Source: CAD feature listing. Evaluate the final solid. Frame: model axes, mm. A direction names the side the tool comes from. Give positions to 0.01 mm unless a question says otherwise; leave off trailing zeros. Order: outer loops, then holes, each group sorted by start corner. A loop starts at its lowest first (then second) coordinate and runs counter-clockwise, first axis right, second up. Notation, with made-up numbers: M -39,64.25 L -4,64.25 A25 ccw -4,88.25 Z; hole C -1.75,-25 d7. An arc over 180 degrees is marked long. Answer in a Markdown table with one row per item. Add a question column.
(1) Section query A-A, the plane z = 3. Return loops of the section in (x, y) (3 decimals), plus the area to 3 significant figures.
(2) Section query C-C, the plane z = 20.5. Return loops of the section in (x, y) (3 decimals), plus the area to 3 significant figures.
(3) Mould query, pull axis X, two halves, no side actions, for faces 5 (the face through (-63.5, 0, 13)), 6 (the face through (-26.261, 19.547, 22.471)), 7 (the face through (0, 17, -25.4)), 8 (the face through (76.2, 0, 25)). Classes: pulls with the +X half, pulls with the -X half, needs draft (parallel to the pull), parting line crosses it, or undercut.
(4) Section query D-D, the plane x = 36. Return loops of the section in (y, z).
(5) Section query B-B, the plane z = 30. Count the separate pieces of the cut face and the enclosed holes in it, plus the area to 3 significant figures.
(6) Set-up query: faces 1 (the face through (-60.324, 0.332, 12.878)), 2 (the face through (-21.368, 21.274, 30.185)), 3 (the face through (35.67, -12.6, 28.53)), 4 (the face through (-35.67, 12.6, 28.53)). Return all of +Z, -Z, +X, -X, +Y, -Y with unobstructed straight access to the full face (end or side cutting, diameter ignored); none if empty.
(7) Material intervals for line 1 along Z through (x, y) = (-64.5, 15) (3 decimals); line 2 along X through (y, z) = (-20, 29); line 3 along X through (y, z) = (19, 10.5), sorted ascending.
(8) Pin query (flat end, axial travel): P1, Ø2.5, axis at x = 24.4, y = 20.32, coming from the +Z side; P2, Ø6.5, axis at x = 24.4, y = -20.32, coming from the -Z side; P3, Ø5, axis at x = -8.5, z = -5.5, coming from the -Y side. Return the tip coordinate at first contact, or that it passes through.
from build123d import *

# Parameters (mm, degrees)
SKETCH1_W                        = 152.4
SKETCH1_H                        = 63.5
BOSS_EXTRUDE1_DEPTH              = 25.4
BOSS_EXTRUDE2_DEPTH              = 9.525
BOSS_EXTRUDE3_DEPTH              = 6.35
CUT_EXTRUDE1_DEPTH               = 87.36933773
SKETCH5_R                        = 25.4
BOSS_EXTRUDE4_DEPTH              = 25.4
CUT_EXTRUDE2_DEPTH               = 103.242887894
F_7_16_20_TAPPED_HOLE2_OUTLINE_W = 4.96062
F_7_16_20_TAPPED_HOLE2_OUTLINE_H = 9.52526547
SKETCH13_R                       = 3.175
CUT_EXTRUDE3_DEPTH               = 3.175
F_10_32_TAPPED_HOLE1_D           = 4.0386
F_10_32_TAPPED_HOLE1_DEPTH       = 12.0396
F_10_32_TAPPED_HOLE1_TIP         = 1.213317848
FILLET1_R                        = 3.175
SKETCH16_W                       = 12.7
SKETCH16_H                       = 6.35
CUT_EXTRUDE4_DEPTH               = 106.159144277
CHAMFER1_SIZE                    = 9.525
CHAMFER2_SIZE                    = 9.525


# Read off the part's stored shape, not the designer's step: 7/16-20 Tapped Hole2
with BuildPart() as part:
    # Sketch1 → Boss-Extrude1 (new body)
    with BuildSketch(Plane.XY):
        Rectangle(SKETCH1_W, SKETCH1_H)
    extrude(amount=BOSS_EXTRUDE1_DEPTH)

    # Sketch2 → Boss-Extrude2 (add)
    with BuildSketch(Plane.XY.offset(25.4)):
        with BuildLine():
            Line((-57.15, 31.75), (-76.2, 31.75))
            Line((-76.2, 31.75), (-76.2, -31.75))
            Line((-76.2, -31.75), (-57.15, -31.75))
            ThreePointArc((-57.15, -31.75), (-65.65738686, 0), (-57.15, 31.75))
        make_face()
        with BuildLine():
            Line((57.15, 31.75), (76.2, 31.75))
            Line((76.2, 31.75), (76.2, -31.75))
            Line((76.2, -31.75), (57.15, -31.75))
            ThreePointArc((57.15, -31.75), (65.65738686, 0), (57.15, 31.75))
        make_face()
    extrude(amount=BOSS_EXTRUDE2_DEPTH)

    # Sketch3 → Boss-Extrude3 (add)
    with BuildSketch(Plane.XY.offset(25.4)):
        with BuildLine():
            ThreePointArc((0, 31.75), (-6.499067792, 31.272316494), (-12.858450657, 29.849532861))
            ThreePointArc((-12.858450657, 29.849532861), (-20.139715933, 27.86213325), (-27.51768912, 26.270878114))
            ThreePointArc((-27.51768912, 26.270878114), (-29.380205079, 25.48503317), (-30.748971212, 23.997418552))
            ThreePointArc((-30.748971212, 23.997418552), (-35.717260564, 12.431977761), (-37.689378393, 0))
            ThreePointArc((-37.689378393, 0), (-35.717260564, -12.431977761), (-30.748971212, -23.997418552))
            ThreePointArc((-30.748971212, -23.997418552), (-29.380205079, -25.48503317), (-27.51768912, -26.270878114))
            ThreePointArc((-27.51768912, -26.270878114), (-20.139715933, -27.86213325), (-12.858450657, -29.849532861))
            ThreePointArc((-12.858450657, -29.849532861), (-6.499067792, -31.272316494), (0, -31.75))
            ThreePointArc((0, -31.75), (6.499067792, -31.272316494), (12.858450657, -29.849532861))
            ThreePointArc((12.858450657, -29.849532861), (20.139715933, -27.86213325), (27.51768912, -26.270878114))
            ThreePointArc((27.51768912, -26.270878114), (29.380205079, -25.48503317), (30.748971212, -23.997418552))
            ThreePointArc((30.748971212, -23.997418552), (35.717260564, -12.431977761), (37.689378393, 0))
            ThreePointArc((37.689378393, 0), (35.717260564, 12.431977761), (30.748971212, 23.997418552))
            ThreePointArc((30.748971212, 23.997418552), (29.380205079, 25.48503317), (27.51768912, 26.270878114))
            ThreePointArc((27.51768912, 26.270878114), (20.139715933, 27.86213325), (12.858450657, 29.849532861))
            ThreePointArc((12.858450657, 29.849532861), (6.499067792, 31.272316494), (0, 31.75))
        make_face()
    extrude(amount=BOSS_EXTRUDE3_DEPTH)

    # Sketch4 → Cut-Extrude1 (cut, through all)
    with BuildSketch(Plane.XY.offset(25.4)):
        with BuildLine():
            ThreePointArc((-55.733032799, 23.085378057), (-60.325, 0), (-55.733032799, -23.085378057))
            ThreePointArc((-55.733032799, -23.085378057), (-47.436357972, -26.521973293), (-43.999762736, -18.225298466))
            ThreePointArc((-43.999762736, -18.225298466), (-47.625, 0), (-43.999762736, 18.225298466))
            ThreePointArc((-43.999762736, 18.225298466), (-47.436357972, 26.521973293), (-55.733032799, 23.085378057))
        make_face()
    cut_extrude1 = extrude(amount=-CUT_EXTRUDE1_DEPTH, mode=Mode.SUBTRACT)

    # Mirror1: Cut-Extrude1 across plane
    add(cut_extrude1.mirror(Plane(origin=(0, 0, 0), x_dir=(0, 0, 1), z_dir=(1, 0, 0))), mode=Mode.SUBTRACT)

    # Sketch5 → Boss-Extrude4 (add)
    with BuildSketch(Plane(origin=(0, 0, 0), x_dir=(-1, 0, 0), z_dir=(0, 0, -1))):
        with Locations(Location((0, 0, 0), (0, 0, 180))):
            Circle(SKETCH5_R)
    extrude(amount=BOSS_EXTRUDE4_DEPTH)

    # Sketch6 → Cut-Extrude2 (cut, through all)
    with BuildSketch(Plane(origin=(0, 0, -25.4), x_dir=(-1, 0, 0), z_dir=(0, 0, -1))):
        Polygon((9.165435523, -15.875), (18.330871047, 0), (9.165435523, 15.875), (-9.165435523, 15.875), (-18.330871047, 0), (-9.165435523, -15.875), align=None)
    extrude(amount=-CUT_EXTRUDE2_DEPTH, mode=Mode.SUBTRACT)

    # 7/16-20 Tapped Hole2 outline → 7/16-20 Tapped Hole2 (revolve, cut)
    with BuildSketch(Plane(origin=(0.052782238, -0.091421518, -15.875), x_dir=(0.5000000000000003, -0.8660254037844385, 0), z_dir=(0, 0, 1))):
        with Locations((2.48031, 20.637632735)):
            Rectangle(F_7_16_20_TAPPED_HOLE2_OUTLINE_W, F_7_16_20_TAPPED_HOLE2_OUTLINE_H)
    f_7_16_20_tapped_hole2 = revolve(axis=Axis((0.052782238, -0.091421518, -15.875), (0.8660254037844385, 0.5000000000000003, 0)), mode=Mode.SUBTRACT)

    # Mirror6: 7/16-20 Tapped Hole2 across plane
    add(f_7_16_20_tapped_hole2.mirror(Plane(origin=(0, 0, 0), x_dir=(0, 0, 1), z_dir=(1, 0, 0))), mode=Mode.SUBTRACT)

    # Sketch13 → Cut-Extrude3 (cut)
    with BuildSketch(Plane.XY.offset(31.75)):
        with Locations((-24.395903345, 20.32)):
            Circle(SKETCH13_R)
        with Locations((24.395903345, 20.32)):
            Circle(SKETCH13_R)
        with Locations((24.395903345, -20.32)):
            Circle(SKETCH13_R)
        with Locations((-24.395903345, -20.32)):
            Circle(SKETCH13_R)
    extrude(amount=-CUT_EXTRUDE3_DEPTH, mode=Mode.SUBTRACT)

    # #10-32 Tapped Hole1
    with Locations(Plane.XY.offset(28.575)):
        with Locations((-24.395903345, 20.32), (24.395903345, 20.32), (24.395903345, -20.32), (-24.395903345, -20.32)):
            Hole(F_10_32_TAPPED_HOLE1_D / 2, depth=F_10_32_TAPPED_HOLE1_DEPTH)
            with Locations((0, 0, -(F_10_32_TAPPED_HOLE1_DEPTH + F_10_32_TAPPED_HOLE1_TIP / 2))):  # 118° drill point
                Cone(0, F_10_32_TAPPED_HOLE1_D / 2, F_10_32_TAPPED_HOLE1_TIP, mode=Mode.SUBTRACT)

    # Fillet1
    fillet1_edges = [part.edges().sort_by_distance(p)[0] for p in [
        (-25.4, 0, 0),
    ]]
    fillet(fillet1_edges, radius=FILLET1_R)

    # Sketch16 → Cut-Extrude4 (cut, through all)
    with BuildSketch(Plane(origin=(0, 31.75, 0), x_dir=(1, 0, 0), z_dir=(0, 1, 0))):
        with Locations((69.85, -12.7)):
            Rectangle(SKETCH16_W, SKETCH16_H)
        with Locations((-69.85, -12.7)):
            Rectangle(SKETCH16_W, SKETCH16_H)
    extrude(amount=-CUT_EXTRUDE4_DEPTH, mode=Mode.SUBTRACT)

    # Chamfer1
    chamfer1_edges = [part.edges().sort_by_distance(p)[0] for p in [
        (-76.2, 31.75, 4.7625),
        (76.2, 31.75, 4.7625),
        (-76.2, 31.75, 25.4),
        (76.2, 31.75, 25.4),
    ]]
    chamfer(chamfer1_edges, length=CHAMFER1_SIZE)

    # Chamfer2
    chamfer2_edges = [part.edges().sort_by_distance(p)[0] for p in [
        (76.2, -31.75, 4.7625),
        (-76.2, -31.75, 4.7625),
        (76.2, -31.75, 25.4),
        (-76.2, -31.75, 25.4),
    ]]
    chamfer(chamfer2_edges, length=CHAMFER2_SIZE)


solid = part.part
Values follow:
| question | item | result |
|---|---|---|
| 1 | outline | M -76.2,-22.225 L -66.675,-31.75 L 66.675,-31.75 L 76.2,-22.225 L 76.2,22.225 L 66.675,31.75 L -66.675,31.75 L -76.2,22.225 Z; hole M -55.733,-23.085 A6.35 ccw -44,-18.225 A47.625 cw -44,18.225 A6.35 ccw -55.733,23.085 A60.325 ccw Z; hole M -18.331,0 L -9.165,-15.875 L 9.165,-15.875 L 18.331,0 L 9.165,15.875 L -9.165,15.875 Z; hole M 44,-18.225 A6.35 ccw 55.733,-23.085 A60.325 ccw 55.733,23.085 A6.35 ccw 44,18.225 A47.625 cw Z |
| 1 | area | 7,290 mm² |
| 2 | outline | M -76.2,-22.225 L -66.675,-31.75 L 66.675,-31.75 L 76.2,-22.225 L 76.2,22.225 L 66.675,31.75 L -66.675,31.75 L -76.2,22.225 Z; hole M -55.733,-23.085 A6.35 ccw -44,-18.225 A47.625 cw -44,18.225 A6.35 ccw -55.733,23.085 A60.325 ccw Z; hole C -24.396,-20.32 d4.039; hole C -24.396,20.32 d4.039; hole M -18.331,0 L -9.165,-15.875 L 9.165,-15.875 L 18.331,0 L 9.165,15.875 L -9.165,15.875 Z; hole C 24.396,-20.32 d4.039; hole C 24.396,20.32 d4.039; hole M 44,-18.225 A6.35 ccw 55.733,-23.085 A60.325 ccw 55.733,23.085 A6.35 ccw 44,18.225 A47.625 cw Z |
| 2 | area | 7,240 mm² |
| 3 | face 5 | pulls with the -X half |
| 3 | face 6 | undercut |
| 3 | face 7 | needs draft |
| 3 | face 8 | pulls with the +X half |
| 4 | outline | M -31.75,0 L 31.75,0 L 31.75,25.4 L 11.41,25.4 L 11.41,31.75 L -11.41,31.75 L -11.41,25.4 L -31.75,25.4 Z |
| 5 | separate pieces | 3 |
| 5 | enclosed holes | 5 |
| 5 | area | 4,510 mm² |
| 6 | face 1 | +Z, -Z |
| 6 | face 2 | +Z |
| 6 | face 3 | +Z, -Y |
| 6 | face 4 | +Z, +Y |
| 7 | line 1 | z = 0 to 9.525, 15.875 to 34.925 |
| 7 | line 2 | x = -76.2 to -62.43, -32.86 to -27.55, -21.24 to 21.24, 27.55 to 32.86, 62.43 to 76.2 |
| 7 | line 3 | x = -63.5 to -57.25, -43.74 to 43.74, 57.25 to 63.5 |
| 8 | P1 | stops at z = 16.08 |
| 8 | P2 | stops at z = 0 |
| 8 | P3 | stops at y = -24.68 |
